Autodesk Inventor part; units mm, degrees
ref_plane "YZ Plane" through (0, 0, 0) normal (1, 0, 0) x (0, 1, 0)
ref_plane "XZ Plane" through (0, 0, 0) normal (0, 1, 0) x (-1, 0, 0)
ref_plane "XY Plane" through (0, 0, 0) normal (0, 0, 1) x (1, 0, 0)
sketch "Sketch1" plane through (0, 0, 0) normal (0, 0, 1) x (1, 0, 0)
  arc A0 (0, 7.5) -> (-7.5, 0) centre (0, 0) ccw
  line L0 (-7.5, 0) -> (-19.5, 0)
  line L1 (-19.5, 0) -> (-19.5, 3)
  arc A1 (0, 10.5) -> (-9.6234, 4.2) centre (0, 0) ccw
  line L2 (-19.5, 3) -> (-11.4564, 3)
  line L3 (0, 10.5) -> (0, 7.5)
  arc A2 (-11.4564, 3) -> (-9.6234, 4.2) centre (-11.4564, 5) ccw
  point P0 (-10.0623, 3)
  dimension "d0" = 15
  dimension "d1" = 12
  dimension "d2" = 3
  dimension "d3" = 3
  dimension "d4" = 2
extrude "Extrusion1" add sketch "Sketch1" along normal mid plane 15
sketch "Sketch2" plane through (-19.5, 3, 7.5) normal (0, 1, 0) x (1, 0, 0)
  line L0 (-3.9, 7.5) -> (23.4, 7.5)
  circle A0 centre (5, 7.5) radius 2
  line L1 (0, 15) -> (0, 0)
  point P0 (19.5, 7.5)
  dimension "d7" = 4
  dimension "d8" = 5
extrude "Extrusion2" cut sketch "Sketch2" against normal blind 15
chamfer "Chamfer1" distance 1 angle 45 1 edges at (-16.5, 3, 0)
mirror "Mirror1" about plane through (0, 7.5, 0) normal (1, 0, 0) of "Extrusion1", "Extrusion2", "Chamfer1"
properties part number "CableWallMount"
Can you work these out from the model? Positions are in its coordinate system, mm. A direction names the side the tool comes from. Coordinates: 2 decimals unless noted, no trailing zeros. Loops run counter-clockwise (first coordinate to the right, second up) from the corner with the lowest first, then second, coordinate; pieces in that order, holes last.
1) I need wall thicknesses on probe 1 along Z at (x, y) = (14.5, 1.55); probe 2 along X at (y, z) = (0.75, -0.25); probe 3 along Y at (x, z) = (12, 1.75). Which ranges of each line are inside material? Lowest first, please.
2) Imagine slicing it at A-A on z = 0. List the corners of the cut face in (x, y) for me.
3) Which directions (+Z, -Z, +X, -X, +Y, -Y) give clear straight access to the entire face, cutting with the end or side of a thin tool? Please do faces 1 (the flat face through (17, 3, -2)), 2 (the cylindrical face through (-16.1, 1, 1.2)).
4) Thinking about a two-plate mould opening in Z: for faces 3 (the flat face through (-17, 3, -2)), 4 (the cylindrical face through (16.1, 1, -1.2)), 5 (the flat face through (0, 8, -7.5)), which applies, pulls with the +Z half, pulls with the -Z half, needs draft (parallel to the pull), parting line crosses it, or undercut?
5) Imagine slicing it at D-D on x = -6. List the corners of the cut face in (y, z) for me, plus the area to 3 significant figures.
6) Imagine slicing it at B-B on x = -14.5. List the corners of the cut face in (y, z) for me, plus the area to 3 significant figures.
7) Imagine slicing it at C-C on y = 6. List the corners of the cut face in (x, z) for me.
8) For pin 1 (2 mm diameter, centred on x = 9, z = -2.5, fed in from +Y); pin 2 (6.5 mm diameter, centred on x = -15.5, z = 2, fed in from +Y); pin 3 (1.5 mm diameter, centred on y = 6, z = -5, fed in from -X), each with a flat end and sliding along its axis, tell me the tip position at first contact or that it passes through.
Completed:
1. probe 1: z = -7.5 to -2, 2 to 7.5
1. probe 2: x = -19.5 to -16.48, -12.52 to -7.46, 7.46 to 12.52, 16.48 to 19.5
1. probe 3: y = 0 to 3
2. outline: (-19.5, 0) - (-16.5, 0) - (-16.5, 2) - (-17.5, 3) - (-19.5, 3) - close; (-12.5, 0) - (-7.5, 0) arc R7.5 cw to (7.5, 0) - (12.5, 0) - (12.5, 2) - (11.5, 3) - (11.46, 3) arc R2 cw to (9.62, 4.2) arc R10.5 ccw to (0, 10.5) arc R10.5 ccw to (-9.62, 4.2) arc R2 cw to (-11.46, 3) - (-11.5, 3) - (-12.5, 2) - close; (16.5, 0) - (19.5, 0) - (19.5, 3) - (17.5, 3) - (16.5, 2) - close
3. face 1: +Z, -Z, +X, +Y
3. face 2: +Y, -Y
4. face 3: needs draft
4. face 4: undercut
4. face 5: pulls with the -Z half
5. outline: (4.5, -7.5) - (8.62, -7.5) - (8.62, 7.5) - (4.5, 7.5) - close
5. area: 61.8 mm2
6. outline: (0, -7.5) - (3, -7.5) - (3, -3) - (2, -2) - (0, -2) - close; (0, 2) - (2, 2) - (3, 3) - (3, 7.5) - (0, 7.5) - close
6. area: 32.0 mm2
7. outline: (-8.62, -7.5) - (-4.5, -7.5) - (-4.5, 7.5) - (-8.62, 7.5) - close; (4.5, -7.5) - (8.62, -7.5) - (8.62, 7.5) - (4.5, 7.5) - close
8. pin 1: stops at y = 6.8
8. pin 2: stops at y = 3
8. pin 3: stops at x = -9.09
